```python
from build123d import *

# Parameters (mm, degrees)
F1_DEPTH     = 10
F2_R         = 2.5
F3_DEPTH     = 0.5
F4_T4_DEPTH  = 51.44253063
F4_S5_R      = 2.5
F4_T6_DEPTH  = 29
F4_T10_DEPTH = 51.44253063
F4_S11_R     = 2.5
F4_T12_DEPTH = 29


# Not quite as in the source:
# - a fillet or chamfer that OpenCascade refuses, or shapes differently, is made with other operations: its cross-section is extruded or revolved along the edge and cut away or added


with BuildPart() as f1:
    # F0 (on Front) → F1 (new body)
    with BuildSketch(Plane.XZ):
        with BuildLine():
            Line((-18.7246046442, 1.2957563709), (5.805945114, 11.1679169591))
            ThreePointArc((5.805945114, 11.1679169591), (-25.7288225372, 54.1130726963), (-18.7246046442, 1.2957563709))
        make_face()
    extrude(amount=F1_DEPTH)

    # F2 (on face) → F3 (join)
    with BuildSketch(Plane(origin=(-3.0587265768, 0, 7.6003873539), x_dir=(0.9276929694, 0, 0.3733440164), z_dir=(0.3733440164, 0, -0.9276929694))):
        with Locations((-3.6656558802, 4.9999994226)):
            Circle(F2_R)
    extrude(amount=F3_DEPTH)

    # F4: fillet of radius 5 on 2 edges, made by hand


with BuildPart() as f4_tool2:
    # F4_s3 → F4_t4 (new body)
    with BuildSketch(Plane(origin=(-27.2620401847, 0, -10.9714311875), x_dir=(0, 1, 0), z_dir=(0.9276929694, 0, 0.3733440164))):
        with BuildLine():
            ThreePointArc((-5, 8.192783178), (-8.5355339059, 9.657249272), (-10, 13.192783178))
            Line((-10, 13.192783178), (-10, 8.192783178))
            Line((-10, 8.192783178), (-5, 8.192783178))
        make_face()
    extrude(amount=F4_T4_DEPTH)

    # F4_s5 → F4_t6 (cut, symmetric)
    with BuildSketch(Plane(origin=(-3.9947809751, 0, 9.9263147724), x_dir=(0, 1, 0), z_dir=(-0.3733440164, 0, 0.9276929694))):
        with Locations((-4.9999994226, 3.6656558802)):
            Circle(F4_S5_R)
    extrude(amount=F4_T6_DEPTH, both=True, mode=Mode.SUBTRACT)


with BuildPart() as f1_1:
    add(f1.part)

    # F4_t1: cut F4_tool2
    add(f4_tool2.part, mode=Mode.SUBTRACT)


with BuildPart() as f4_tool8:
    # F4_s9 → F4_t10 (new body)
    with BuildSketch(Plane(origin=(-27.2620401847, 0, -10.9714311875), x_dir=(0, 1, 0), z_dir=(0.9276929694, 0, 0.3733440164))):
        with BuildLine():
            ThreePointArc((-5, 8.192783178), (-1.4644660941, 9.657249272), (0, 13.192783178))
            Line((0, 13.192783178), (0, 8.192783178))
            Line((0, 8.192783178), (-5, 8.192783178))
        make_face()
    extrude(amount=F4_T10_DEPTH)

    # F4_s11 → F4_t12 (cut, symmetric)
    with BuildSketch(Plane(origin=(-3.9947809751, 0, 9.9263147724), x_dir=(0, 1, 0), z_dir=(-0.3733440164, 0, 0.9276929694))):
        with Locations((-4.9999994226, 3.6656558802)):
            Circle(F4_S11_R)
    extrude(amount=F4_T12_DEPTH, both=True, mode=Mode.SUBTRACT)


with BuildPart() as f1_2:
    add(f1_1.part)

    # F4_t7: cut F4_tool8
    add(f4_tool8.part, mode=Mode.SUBTRACT)


solid = f1_2.part
```
Geometry: final body of the model. Coordinates: model frame, mm. Give positions to 0.01 mm unless a question says otherwise; leave off trailing zeros. Loops run counter-clockwise (first coordinate to the right, second up) from the corner with the lowest first, then second, coordinate; pieces in that order, holes last. Notation, with made-up numbers: (69, -35.5) -> (85, -35.5) arc R23 ccw to (85, -23.5) -> close; hole circle Ø10 at (29.5, -5.75). An arc over 180 degrees is marked (long way). Use CSV: the item, a comma, the result in double quotes.
(1) Cut plane A-A (y = -6.25). Output: boundary loops of the cut face in (x, z), plus the area to 3 significant figures.
From the geometry:
outline,"(-19.05, 1.34) -> (-8.53, 5.57) -> (-8.28, 4.96) -> (-4.26, 6.58) -> (-4.51, 7.19) -> (6.01, 11.42) arc R27.5 ccw (long way) to start"
area,"2,310 mm^2"
(2) Cut plane C-C (x = -32.5). Output: boundary loops of the cut face in (y, z), plus the area to 3 significant figures.
From the geometry:
outline,"(-10, 7.02) -> (0, 7.02) -> (0, 50.19) -> (-10, 50.19) -> close"
area,"432 mm^2"
(3) First-contact query: P1, Ø3, axis at x = -30, y = -9, coming from the -Z side; P2, Ø4, axis at y = -3.5, z = 47, coming from the +X side; P3, Ø4, axis at y = -5.5, z = 10.5, coming from the -X side. Flat tips, straight axial feed; report the tip coordinate or a pass-through.
From the geometry:
P1,"z = 4.39"
P2,"x = 6.61"
P3,"x = -37.76"
(4) Cut plane D-D (y = -1.75). Output: boundary loops of the cut face in (x, z).
From the geometry:
outline,"(-21.01, 1.67) -> (7.2, 13.02) arc R27.5 ccw (long way) to start"
(5) Cut plane B-B (z = 53.5). Output: boundary loops of the cut face in (x, y), plus the area to 3 significant figures.
From the geometry:
outline,"(-27.14, -10) -> (-3.79, -10) -> (-3.79, 0) -> (-27.14, 0) -> close"
area,"234 mm^2"
(6) Ray query, line 1 along X through (y, z) = (-6.75, 28); line 2 along X through (y, z) = (-9, 48); line 3 along Z through (x, y) = (-36, -1.75). Return the intervals inside material, ascending. Write a range as [from, to].
From the geometry:
line 1,"[-42.96, 12.03]"
line 2,"[-34.95, 4.03]"
line 3,"[10.31, 46.89]"
